Geometry check sheet. Reference: the model listing, model coordinates, mm. Face numbers are marked on the shaded views. A direction names the side the tool comes from. Coordinates: 2 decimals unless noted, no trailing zeros. Write each loop counter-clockwise with the first axis right and the second up, starting at its lowest first coordinate (ties: lowest second). Pieces come first, ordered by that corner, then holes.
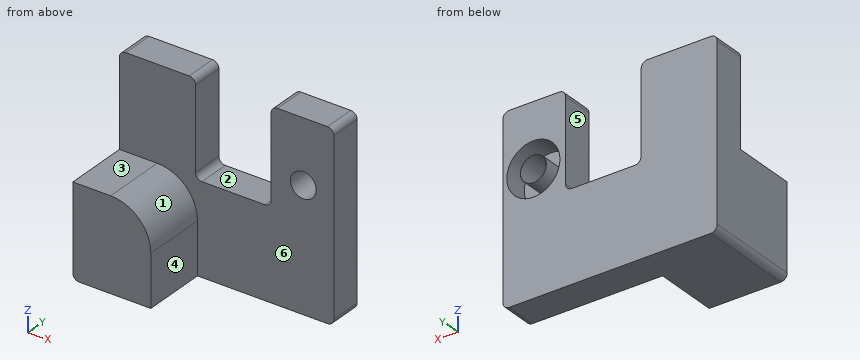
from build123d import *

# Parameters (mm, degrees)
SKETCH1_R           = 2.032
BOSS_EXTRUDE1_DEPTH = 5.08
FILLET2_R           = 1
SKETCH4_R           = 4.191
CUT_EXTRUDE3_DEPTH  = 3.81
SKETCH5_R           = 2.0574
SKETCH5_R_2         = 2.032
BOSS_EXTRUDE2_DEPTH = 3.81
BOSS_EXTRUDE3_DEPTH = 10.16


with BuildPart() as part:
    # Sketch1 → Boss-Extrude1 (new body)
    with BuildSketch(Plane(origin=(0, 0, 0), x_dir=(1, 0, 0), z_dir=(0, 1, 0))):
        Polygon((0, 29.21), (0, 0), (12.022666667, 0), (12.022666667, 14.986), (23.960666667, 14.986), (23.960666667, 0), (33.866666667, 0), (33.866666667, 29.21), align=None)
        with Locations((29.040666667, 10)):
            Circle(SKETCH1_R, mode=Mode.SUBTRACT)
    extrude(amount=BOSS_EXTRUDE1_DEPTH)

    # Fillet2
    fillet2_edges = [part.edges().sort_by_distance(p)[0] for p in [
        (23.960666667, 2.54, -14.986),
        (12.022666667, 2.54, -14.986),
        (12.022666667, 2.54, 0),
        (0, 2.54, 0),
        (0, 2.54, -29.21),
        (33.866666667, 2.54, -29.21),
        (33.866666667, 2.54, 0),
        (23.960666667, 2.54, 0),
    ]]
    fillet(fillet2_edges, radius=FILLET2_R)

    # Sketch4 → Cut-Extrude3 (cut)
    with BuildSketch(Plane(origin=(0, 5.08, 0), x_dir=(1, 0, 0), z_dir=(0, 1, 0))):
        with Locations((29.040666667, 10)):
            Circle(SKETCH4_R)
    extrude(amount=-CUT_EXTRUDE3_DEPTH, mode=Mode.SUBTRACT)

    # Sketch5 → Boss-Extrude2 (add)
    with BuildSketch(Plane(origin=(0, 1.27, 0), x_dir=(1, 0, 0), z_dir=(0, 1, 0))):
        with Locations((29.040666667, 10)):
            Circle(SKETCH5_R)
        with Locations((29.040666667, 10)):
            Circle(SKETCH5_R_2, mode=Mode.SUBTRACT)
    extrude(amount=BOSS_EXTRUDE2_DEPTH)

    # Sketch6 → Boss-Extrude3 (add)
    with BuildSketch(Plane.XZ):
        with BuildLine():
            Line((1, -29.21), (12.315559885, -29.21))
            Line((12.315559885, -29.21), (12.315559885, -21.043106781))
            ThreePointArc((12.315559885, -21.043106781), (10.455687946, -16.552978721), (5.965559885, -14.693106781))
            Line((5.965559885, -14.693106781), (0, -14.693106781))
            Line((0, -14.693106781), (0, -28.21))
            ThreePointArc((0, -28.21), (0.292893219, -28.917106781), (1, -29.21))
        make_face()
    extrude(amount=BOSS_EXTRUDE3_DEPTH)


solid = part.part
1. Thickness scan on line 1 along Y through (x, z) = (14, -25); line 2 along X through (y, z) = (0.5, -8.75); line 3 along X through (y, z) = (-9, -24.75). Record the ranges inside material, lowest first.
Computed values:
line 1: y = 0 to 5.08
line 2: x = 0 to 12.02, 23.96 to 27.44, 30.64 to 33.87
line 3: x = 0 to 12.32
2. Draft check along X on the marked faces 1, 2 and 3. Enter one of: released by +X, released by -X, zero draft, split by the parting line, or undercut.
Computed values:
face 1: released by +X
face 2: undercut
face 3: zero draft
3. Sectioned sample at B-B, the plane z = -10. Give the number of separate pieces and of enclosed holes in the cut face, and give its area (3 significant figures).
Computed values:
separate pieces: 3
enclosed holes: 0
area: 74.5 mm2
4. Gauge pin test, flat ends, axial feed: pin 1 Ø2.5 at (y, z) = (-6, -26.5) entering from +X; pin 2 Ø5 at (x, z) = (12, -10.5) entering from -Y; pin 3 Ø5 at (x, y) = (3, -5) entering from +Z. Record the tip position at first contact, or that the pin passes through.
Computed values:
pin 1: stops at x = 12.32
pin 2: stops at y = 0
pin 3: stops at z = -14.69
5. Sectioned sample at D-D, the plane y = -7. Record the boundary of the cut face in (x, z).
Computed values:
outline: (0, -28.21) arc R1 ccw to (1, -29.21) - (12.32, -29.21) - (12.32, -21.04) arc R6.35 ccw to (5.97, -14.69) - (0, -14.69) - close
6. Access from +Z, -Z, +X, -X, +Y, -Y to the whole of each face (thin tool, end or side, straight path). Record for the marked faces 4, 5 and 6.
Computed values:
face 4: +Z, -Z, +X, -Y
face 5: +Z, +Y, -Y
face 6: +Z, +X, -Y
7. Sectioned sample at A-A, the plane y = 2.75. Record the boundary of the cut face in (x, z), and give its area (3 significant figures).
Computed values:
outline: (0, -28.21) arc R1 ccw to (1, -29.21) - (32.87, -29.21) arc R1 ccw to (33.87, -28.21) - (33.87, -1) arc R1 ccw to (32.87, 0) - (24.96, 0) arc R1 ccw to (23.96, -1) - (23.96, -13.99) arc R1 cw to (22.96, -14.99) - (13.02, -14.99) arc R1 cw to (12.02, -13.99) - (12.02, -1) arc R1 ccw to (11.02, 0) - (1, 0) arc R1 ccw to (0, -1) - close; circle Ø4.11 at (29.04, -10); hole circle Ø8.38 at (29.04, -10); hole circle Ø4.06 at (29.04, -10)
area: 755 mm2
